Could you check a few things on this model? Use its own coordinates, in mm. A direction names the side the tool comes from. Give positions to 0.01 mm unless a question says otherwise; leave off trailing zeros. Write each loop counter-clockwise with the first axis right and the second up, starting at its lowest first coordinate (ties: lowest second). Pieces come first, ordered by that corner, then holes. Notation, with made-up numbers: (-25.5, 68.5) - (11.5, 68.5) arc R23 ccw to (11.5, 106.5) - close; hole circle Ø8 at (50.5, -2). An arc over 180 degrees is marked (long way). Write item = value, one per line.
from build123d import *

# Parameters (mm, degrees)
F1_W     = 98.493554
F1_H     = 68.641916
F2_DEPTH = 3.81
F0_W     = 98.33321
F0_H     = 50.405774
F3_DEPTH = 3.81
F4_R     = 1.27
F5_R     = 1.27


with BuildPart() as f2:
    # F1 (on Front) → F2 (new body)
    with BuildSketch(Plane.XZ):
        with Locations((2.817497, 34.320958)):
            Rectangle(F1_W, F1_H)
    extrude(amount=F2_DEPTH)

    # F0 (on Top) → F3 (join)
    with BuildSketch(Plane.XY):
        with Locations((2.568968, -25.202887)):
            Rectangle(F0_W, F0_H)
    extrude(amount=F3_DEPTH)

    # F4
    f4_edges = [f2.edges().sort_by_distance(p)[0] for p in [
        (-46.42928, -3.81, 36.225958),
        (2.817497, -3.81, 68.641916),
        (52.064274, -3.81, 34.320958),
    ]]
    fillet(f4_edges, radius=F4_R)

    # F5
    f5_edges = [f2.edges().sort_by_distance(p)[0] for p in [
        (2.568968, -50.405774, 3.81),
        (51.735573, -26.899166, 3.81),
        (-46.597637, -25.202887, 3.81),
    ]]
    fillet(f5_edges, radius=F5_R)


solid = f2.part
1. Which directions (+Z, -Z, +X, -X, +Y, -Y) give clear straight access to the entire face, cutting with the end or side of a thin tool? Please do faces 1 (the face through (2, -25, 0)), 2 (the face through (51.736, -27, 1)), 3 (the face through (-46.429, -1, 35)), 4 (the face through (2, -26, 3.81)), 5 (the face through (2, 0, 34)).
Filled sheet:
face_1 = -Z, +X, -X, +Y, -Y
face_2 = +Z, -Z, +X, -Y
face_3 = +Z, -X, +Y, -Y
face_4 = +Z, +X, -X, -Y
face_5 = +Z, -Z, +X, -X, +Y
2. If we section it at C-C, the plane y = -34: Please give me the cut outline in (x, z).
Filled sheet:
outline = (-46.6, 0) - (51.74, 0) - (51.74, 2.54) arc R1.27 ccw to (50.47, 3.81) - (-45.33, 3.81) arc R1.27 ccw to (-46.6, 2.54) - close
3. I need wall thicknesses on line 1 (Z direction, x = 1, y = -20.5); line 2 (Y direction, x = -42, z = 40); line 3 (Z direction, x = -12, y = -3). Which ranges of each line are inside material? Lowest first, please.
Filled sheet:
line_1 = 0 to 3.81
line_2 = -3.81 to 0
line_3 = 0 to 68.56
4. If we section it at B-B, the plane z = 26: Please give me the cut outline in (x, y), and give its area (3 significant figures).
Filled sheet:
outline = (-46.43, -2.54) arc R1.27 ccw to (-45.16, -3.81) - (50.79, -3.81) arc R1.27 ccw to (52.06, -2.54) - (52.06, 0) - (-46.43, 0) - close
area = 375 mm2
5. If we section it at A-A, the plane x = 17.5: Please give me the cut outline in (y, z), and give its area (3 significant figures).
Filled sheet:
outline = (-50.41, 0) - (0, 0) - (0, 68.64) - (-2.54, 68.64) arc R1.27 ccw to (-3.81, 67.37) - (-3.81, 3.81) - (-49.14, 3.81) arc R1.27 ccw to (-50.41, 2.54) - close
area = 438 mm2
6. For pin 1 (22.5 mm diameter, centred on x = 3, y = -21, fed in from +Z); pin 2 (19 mm diameter, centred on x = -16, z = 44, fed in from -Y); pin 3 (3 mm diameter, centred on y = -1.5, z = 22.5, fed in from -X); pin 4 (4 mm diameter, centred on x = 34, y = -27, fed in from -Z), each with a flat end and sliding along its axis, tell me the tip position at first contact or that it passes through.
Filled sheet:
pin_1 = 3.81
pin_2 = -3.81
pin_3 = -46.43
pin_4 = 0
